Geometry: final body of the model. Coordinates: model frame, mm. Face numbers are marked on the shaded views. A direction names the side the tool comes from. Give positions to 0.01 mm unless a question says otherwise; leave off trailing zeros. Order: outer loops, then holes, each group sorted by start corner. A loop starts at its lowest first (then second) coordinate and runs counter-clockwise, first axis right, second up. Notation, with made-up numbers: (65, 77) -> (111, 77) arc R20 cw to (111, 95) -> close; hole circle Ø11 at (-35, -30.5). An arc over 180 degrees is marked (long way). One line per question, with ' | ' between items.
from build123d import *

# Parameters (mm, degrees)
SKETCH1_R           = 2.855
BOSS_EXTRUDE1_DEPTH = 6.35
SKETCH2_W           = 15
SKETCH2_H           = 8
BOSS_EXTRUDE2_DEPTH = 44.45
SKETCH3_R           = 6
CUT_EXTRUDE1_DEPTH  = 25.4
SKETCH4_R           = 2.855
BOSS_EXTRUDE3_DEPTH = 20.32
SKETCH5_W           = 8
SKETCH5_H           = 6.35
BOSS_EXTRUDE4_DEPTH = 12.7
SKETCH6_W           = 6.812329396
SKETCH6_H           = 8
BOSS_EXTRUDE5_DEPTH = 6.35


with BuildPart() as part:
    # Sketch1 → Boss-Extrude1 (new body)
    with BuildSketch(Plane(origin=(0, 0, 0), x_dir=(1, 0, 0), z_dir=(0, 1, 0))):
        with Locations(Location((0, 0, 0), (0, 0, 270))):
            Circle(SKETCH1_R)
    extrude(amount=BOSS_EXTRUDE1_DEPTH)

    # Sketch2 → Boss-Extrude2 (add)
    with BuildSketch(Plane(origin=(0, 6.35, 0), x_dir=(1, 0, 0), z_dir=(0, 1, 0))):
        Rectangle(SKETCH2_W, SKETCH2_H)
    extrude(amount=BOSS_EXTRUDE2_DEPTH)

    # Sketch3 → Cut-Extrude1 (cut)
    with BuildSketch(Plane.XY.offset(4)):
        with Locations((0, 21.59)):
            Circle(SKETCH3_R)
    extrude(amount=-CUT_EXTRUDE1_DEPTH, mode=Mode.SUBTRACT)

    # Sketch4 → Boss-Extrude3 (add)
    with BuildSketch(Plane(origin=(0, 50.8, 0), x_dir=(1, 0, 0), z_dir=(0, 1, 0))):
        with Locations(Location((0, 0, 0), (0, 0, 270))):
            Circle(SKETCH4_R)
    extrude(amount=BOSS_EXTRUDE3_DEPTH)

    # Sketch5 → Boss-Extrude4 (add)
    with BuildSketch(Plane.ZY.offset(7.5)):
        with Locations((0, 24.765)):
            Rectangle(SKETCH5_W, SKETCH5_H)
    extrude(amount=BOSS_EXTRUDE4_DEPTH)

    # Sketch6 → Boss-Extrude5 (add)
    with BuildSketch(Plane(origin=(0, 27.94, 0), x_dir=(1, 0, 0), z_dir=(0, 1, 0))):
        with Locations((-16.793835302, 0)):
            Rectangle(SKETCH6_W, SKETCH6_H)
    extrude(amount=BOSS_EXTRUDE5_DEPTH)


solid = part.part
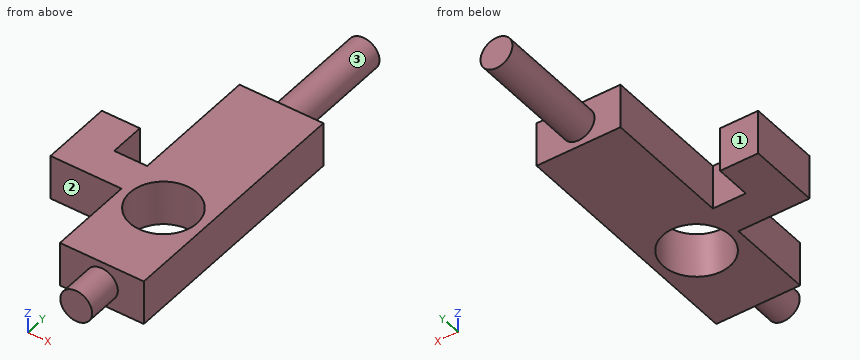
1) Section B-B on x = 0. Return loops of the section in (y, z) (3 decimals).
Check result:
outline: (0, -2.855) -> (6.35, -2.855) -> (6.35, -4) -> (15.59, -4) -> (15.59, 4) -> (6.35, 4) -> (6.35, 2.855) -> (0, 2.855) -> close; (27.59, -4) -> (50.8, -4) -> (50.8, -2.855) -> (71.12, -2.855) -> (71.12, 2.855) -> (50.8, 2.855) -> (50.8, 4) -> (27.59, 4) -> close
2) Set-up query: the marked faces 1, 2 and 3. Return all of +Z, -Z, +X, -X, +Y, -Y with unobstructed straight access to the full face (end or side cutting, diameter ignored); none if empty.
Check result:
face 1: +Z, -Z, -X, +Y | face 2: +Z, -Z, -X, -Y | face 3: +Y
3) Section A-A on y = 33. Return loops of the section in (x, z).
Check result:
outline: (-20.2, -4) -> (-13.39, -4) -> (-13.39, 4) -> (-20.2, 4) -> close; (-7.5, -4) -> (7.5, -4) -> (7.5, 4) -> (-7.5, 4) -> close
4) Section D-D on x = -10.75. Return loops of the section in (y, z).
Check result:
outline: (21.59, -4) -> (27.94, -4) -> (27.94, 4) -> (21.59, 4) -> close
5) Section C-C on z = 0. Return loops of the section in (x, y) (3 decimals).
Check result:
outline: (-20.2, 21.59) -> (-7.5, 21.59) -> (-7.5, 6.35) -> (-2.855, 6.35) -> (-2.855, 0) -> (2.855, 0) -> (2.855, 6.35) -> (7.5, 6.35) -> (7.5, 50.8) -> (2.855, 50.8) -> (2.855, 71.12) -> (-2.855, 71.12) -> (-2.855, 50.8) -> (-7.5, 50.8) -> (-7.5, 27.94) -> (-13.388, 27.94) -> (-13.388, 34.29) -> (-20.2, 34.29) -> close; hole circle Ø12 at (0, 21.59)
6) Contact query for flat-ended pins moving along their axis: pin 1 Ø4 at (y, z) = (62, 0) entering from +X (3 decimals); pin 2 Ø4 at (x, z) = (-12.5, -1.5) entering from -Y; pin 3 Ø2.5 at (y, z) = (16, 0.5) entering from -X. Output: stop coordinate, or through.
Check result:
pin 1: stops at x = 2.855 | pin 2: stops at y = 21.59 | pin 3: stops at x = -7.5
7) Material intervals for probe 1 along X at (y, z) = (29.5, -1.25); probe 2 along Y at (x, z) = (0, 1.5); probe 3 along X at (y, z) = (11.5, 3.5), sorted ascending. Write a range as from..to.
Check result:
probe 1: x = -20.2..-13.39, -7.5..7.5 | probe 2: y = 0..15.59, 27.59..71.12 | probe 3: x = -7.5..7.5
